```python
from build123d import *

# Parameters (mm, degrees)
F0_R     = 12.7
F1_DEPTH = 25.4
F5_D     = 6.35
F5_DEPTH = 12.7
F5_TIP   = 1.9077324654
F7_D     = 6.35
F7_DEPTH = 127
F7_START = 6.3500001
F7_TIP   = 1.9077324654


with BuildPart() as f1:
    # F0 (on Right) → F1 (new body)
    with BuildSketch(Plane.YZ):
        with BuildLine():
            Line((50.8, 50.8), (0, 50.8))
            ThreePointArc((0, 50.8), (-25.4, 25.4), (0, 0))
            Line((0, 0), (50.8, 0))
            Line((50.8, 0), (76.2, -25.4))
            Line((76.2, -25.4), (127, -25.4))
            Line((127, -25.4), (127, 76.2))
            Line((127, 76.2), (76.2, 76.2))
            Line((76.2, 76.2), (50.8, 50.8))
        make_face()
        with Locations((0, 25.4)):
            Circle(F0_R, mode=Mode.SUBTRACT)
    extrude(amount=F1_DEPTH)

    # F2 (on face) → F3 (revolve, cut)
    with BuildSketch(Plane(origin=(0, 127, 0), x_dir=(-1, 0, 0), z_dir=(0, 1, 0))):
        with BuildLine():
            ThreePointArc((-12.7, 50.8), (-17.1901280605, 48.9401280605), (-19.05, 44.45))
            Line((-19.05, 44.45), (-19.05, 6.35))
            ThreePointArc((-19.05, 6.35), (-17.1901280605, 1.8598719395), (-12.7, 0))
            Line((-12.7, 0), (-12.7, 50.8))
        make_face()
    revolve(axis=Axis((12.7, 127, 25.4), (0, 0, -1)), mode=Mode.SUBTRACT)

    # F5
    with Locations(Plane(origin=(0, 127, 0), x_dir=(-1, 0, 0), z_dir=(0, 1, 0))):
        with Locations((-12.7, 63.5), (-12.7, -12.7)):
            Hole(F5_D / 2, depth=F5_DEPTH)
            with Locations((0, 0, -(F5_DEPTH + F5_TIP / 2))):  # 118° drill point
                Cone(0, F5_D / 2, F5_TIP, mode=Mode.SUBTRACT)

    # F7
    # its depths count from where the whole tool has entered the part; down to there all is cleared
    with Locations(Plane(origin=(0, 127, 0), x_dir=(-1, 0, 0), z_dir=(0, 1, 0)).offset(-F7_START)):
        with Locations((-12.7, 24.4230292737)):
            Hole(F7_D / 2, depth=F7_DEPTH)
            with Locations((0, 0, -(F7_DEPTH + F7_TIP / 2))):  # 118° drill point
                Cone(0, F7_D / 2, F7_TIP, mode=Mode.SUBTRACT)


solid = f1.part
```
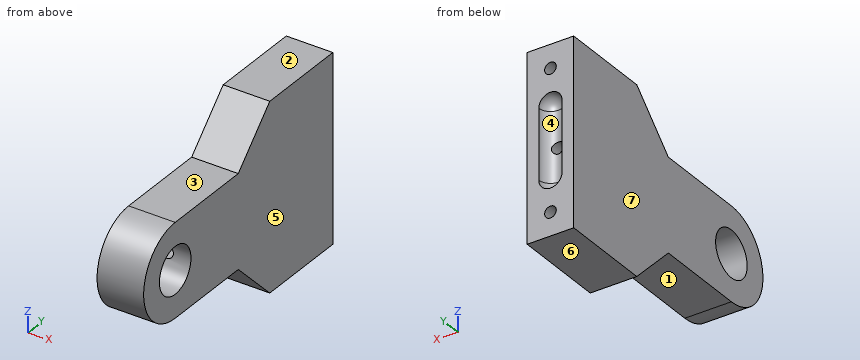
Source: CAD feature listing. Evaluate the final solid. Frame: model axes, mm. Face numbers are marked on the shaded views. A direction names the side the tool comes from. Coordinates: 2 decimals unless noted, no trailing zeros. Loops run counter-clockwise (first coordinate to the right, second up) from the corner with the lowest first, then second, coordinate; pieces in that order, holes last. Notation, with made-up numbers: (32.5, 35) -> (43.5, 35) arc R24 ccw to (43.5, 61) -> close; hole circle Ø8 at (46.25, 1). An arc over 180 degrees is marked (long way). One line per item, written item: value. Start each with the question number.
Q1. Set-up query: the marked faces 1, 2 and 3. Return all of +Z, -Z, +X, -X, +Y, -Y with unobstructed straight access to the full face (end or side cutting, diameter ignored); none if empty.
Q2. Section query C-C, the plane y = 53.5. Return the cut outline in (x, z) (3 decimals).
Q3. Line query: line 1 along Z through (x, y) = (12.7, 118.25) (3 decimals); line 2 along X through (y, z) = (123, 63.5) (3 decimals); line 3 along Z through (x, y) = (12.7, 42). Output: solid intervals per line, ascending.
Q4. Section query D-D, the plane z = -5. Return the cut outline in (x, y).
Q5. Mould query, pull axis X, two halves, no side actions, for the marked faces 4, 5, 6 and 7. Classes: pulls with the +X half, pulls with the -X half, needs draft (parallel to the pull), parting line crosses it, or undercut.
Q6. Section query A-A, the plane y = -2. Return the cut outline in (x, z).
Q7. Section query B-B, the plane z = 46. Return the cut outline in (x, y).
Q8. Contact query for flat-ended pins moving along their axis: P1, Ø7.5, axis at x = 16, y = 30.5, coming from the +Z side; P2, Ø15, axis at y = 0, z = 25.4, coming from the -X side; P3, Ø3, axis at x = 12.5, z = 5, coming from the +Y side; P4, Ø7.5, axis at x = 6.5, y = 18, coming from the -Z side. Output: stop coordinate, or through.
Results:
1. face 1: -Z, +X, -X, -Y
1. face 2: +Z, +X, -X, +Y, -Y
1. face 3: +Z, +X, -X, -Y
2. outline: (0, -2.7) -> (25.4, -2.7) -> (25.4, 53.5) -> (0, 53.5) -> close; hole circle Ø6.35 at (12.7, 24.423)
3. line 1: -25.4 to -15.875, -9.525 to 21.248, 27.598 to 60.325, 66.675 to 76.2
3. line 2: 0 to 9.525, 15.875 to 25.4
3. line 3: 0 to 21.25, 27.6 to 50.8
4. outline: (0, 55.8) -> (25.4, 55.8) -> (25.4, 127) -> (0, 127) -> close
5. face 4: undercut
5. face 5: pulls with the +X half
5. face 6: needs draft
5. face 7: pulls with the -X half
6. outline: (0, 0.08) -> (25.4, 0.08) -> (25.4, 12.86) -> (0, 12.86) -> close; (0, 37.94) -> (25.4, 37.94) -> (25.4, 50.72) -> (0, 50.72) -> close
7. outline: (0, -14.86) -> (25.4, -14.86) -> (25.4, 127) -> (18.86, 127) arc R6.16 cw to (6.54, 127) -> (0, 127) -> close
8. P1: z = 50.8
8. P2: through
8. P3: y = 121.33
8. P4: z = 0
